Autodesk Inventor part; units mm, degrees
ref_plane "YZ Plane" through (0, 0, 0) normal (1, 0, 0) x (0, 1, 0)
ref_plane "XZ Plane" through (0, 0, 0) normal (0, 1, 0) x (-1, 0, 0)
ref_plane "XY Plane" through (0, 0, 0) normal (0, 0, 1) x (1, 0, 0)
sketch "Sketch1" plane through (0, 0, 0) normal (0, 1, 0) x (-1, 0, 0)
  line L0 (5.3777, 6.5934) -> (5.3777, -88.6566)
  line L1 (5.3777, -88.6566) -> (-39.0723, -88.6566)
  line L2 (-39.0723, -88.6566) -> (-39.0723, 6.5934)
  line L3 (-39.0723, 6.5934) -> (5.3777, 6.5934)
  point P0 (0, 0)
  dimension "d0" = 95.25
  dimension "d1" = 44.45
extrude "Extrusion1" add sketch "Sketch1" along normal blind 3.175
sketch "Sketch2" plane through (0, 3.175, 0) normal (0, 1, 0) x (1, 0, 0)
  line L0 (39.0723, 88.6566) -> (-5.3777, 88.6566)
  line L1 (-5.3777, 88.6566) -> (-2.2027, 88.6566)
  line L2 (-2.2027, 88.6566) -> (-2.2027, 85.4816)
  line L3 (-2.2027, 85.4816) -> (-1.9487, 85.4816)
  line L4 (-1.9487, 85.4816) -> (-1.9487, 49.9216)
  line L5 (-1.9487, 49.9216) -> (-2.2027, 49.9216)
  line L6 (-2.2027, 49.9216) -> (-2.2027, 85.4816)
  point P0 (0, 0)
  dimension "d4" = 3.175
  dimension "d5" = 3.175
  dimension "d6" = 0.254
  dimension "d7" = 35.56
  dimension "d8" = 35.56
extrude "Extrusion2" add sketch "Sketch2" along normal blind 0.254
fillet "Fillet1" radius 0.127 2 edges at (-1.9487, 3.429, -67.7016) (-2.2027, 3.429, -67.7016)
sketch "Sketch3" plane through (0, 3.175, 0) normal (0, 1, 0) x (1, 0, 0)
  line L0 (39.0723, -6.5934) -> (39.0723, 88.6566)
  line L1 (39.0723, 88.6566) -> (35.9091, 88.6566)
  line L2 (39.0723, 88.6566) -> (-5.3777, 88.6566)
  line L3 (35.9091, 88.6566) -> (35.9091, 85.4816)
  line L4 (35.9091, 85.4816) -> (35.6551, 85.4816)
  line L5 (35.6551, 85.4816) -> (35.6551, 49.9216)
  line L6 (35.6551, 49.9216) -> (35.9091, 49.9216)
  line L7 (35.9091, 49.9216) -> (35.9091, 85.4816)
  point P0 (0, 0)
  dimension "d12" = 3.175
  dimension "d13" = 0.254
  dimension "d14" = 35.56
  dimension "d15" = 0.254
  dimension "d16" = 35.56
extrude "Extrusion3" add sketch "Sketch3" along normal blind 0.254
fillet "Fillet2" radius 0.127 2 edges at (35.9091, 3.429, -67.7016) (35.6551, 3.429, -67.7016)
sketch "Sketch4" plane through (0, 3.175, 0) normal (0, 1, 0) x (1, 0, 0)
  line L0 (-1.9487, 85.4816) -> (-1.9487, 49.9216)
  line L1 (35.6551, 49.9216) -> (35.6551, 85.4816)
  line L2 (-1.9487, 85.4816) -> (35.6551, 85.4816)
  line L3 (35.6551, 85.4816) -> (35.6551, 85.2276)
  line L4 (35.6551, 85.2276) -> (-1.9487, 85.2276)
  line L5 (-1.9487, 85.2276) -> (-1.9487, 85.4816)
  point P0 (0, 0)
  dimension "d20" = 0.254
extrude "Extrusion4" add sketch "Sketch4" along normal blind 0.254
fillet "Fillet3" radius 0.127 2 edges at (16.8532, 3.429, -85.2276) (16.8532, 3.429, -85.4816)
sketch "Sketch5" plane through (-2.2027, 3.175, -85.4816) normal (-1, 0, 0) x (0, 0, 1)
  point P0 (85.4816, -3.175)
sketch "Sketch6" plane through (0, 3.175, 0) normal (0, 1, 0) x (1, 0, 0)
  line L0 (-2.2027, 85.4816) -> (-1.9487, 85.4816)
  line L1 (-2.2027, 85.4816) -> (-2.4567, 85.4816)
  line L2 (35.6551, 85.4816) -> (-1.9487, 85.4816)
  line L3 (-1.9487, 85.4816) -> (-1.6947, 85.4816)
  line L4 (-1.6947, 85.4816) -> (-1.6947, 117.2316)
  line L5 (-2.2027, 85.4816) -> (-2.2027, 117.2316)
  line L6 (-2.2027, 117.2316) -> (-1.6947, 117.2316)
  point P0 (0, 0)
  dimension "d24" = 0.254
  dimension "d25" = 0.254
  dimension "d26" = 31.75
extrude "Extrusion5" add sketch "Sketch6" along normal blind 0.508
fillet "Fillet4" radius 0.127 1 edges at (-1.9487, 3.683, -85.4816)
sketch "Sketch7" plane through (0, 3.683, 0) normal (0, 1, 0) x (1, 0, 0)
  line L0 (-2.2027, 117.2316) -> (-2.2027, 88.6566)
  line L1 (-2.2027, 117.2316) -> (-2.2027, 114.0566)
  line L2 (-2.2027, 114.0566) -> (-1.6947, 114.0566)
  line L3 (-1.6947, 85.6086) -> (-1.6947, 117.2316)
  line L4 (-2.2027, 114.0566) -> (-2.2027, 113.8026)
  line L5 (-2.2027, 113.8026) -> (-1.6947, 113.8026)
  line L6 (-1.6947, 113.8026) -> (-1.6947, 114.0566)
  point P0 (0, 0)
  dimension "d30" = 3.175
  dimension "d31" = 0.254
extrude "Extrusion6" cut sketch "Sketch7" against normal blind 0.254
sketch "Sketch8" plane through (0, 3.683, 0) normal (0, 1, 0) x (1, 0, 0)
  line L0 (-1.6947, 113.8026) -> (-2.2027, 113.8026)
  line L1 (-2.2027, 113.8026) -> (-2.2027, 107.4526)
  line L2 (-2.2027, 117.2316) -> (-2.2027, 88.6566)
  line L3 (-2.2027, 107.4526) -> (-1.6947, 107.4526)
  line L4 (-1.6947, 88.6566) -> (-1.6947, 117.2316)
  line L5 (-2.2027, 107.4526) -> (-2.2027, 107.1986)
  line L6 (-2.2027, 107.1986) -> (-1.6947, 107.1986)
  line L7 (-1.6947, 107.4526) -> (-1.6947, 107.1986)
  line L8 (-2.2027, 107.4526) -> (-1.6947, 107.4526)
  line L9 (-1.6947, 107.1986) -> (-1.6947, 107.4526)
  line L10 (-2.2027, 107.4526) -> (-2.2027, 107.1986)
  line L11 (-2.2027, 107.1986) -> (-1.6947, 107.1986)
  point P0 (0, 0)
  dimension "d34" = 6.35
  dimension "d35" = 0.254
extrude "Extrusion7" cut sketch "Sketch8" against normal blind 0.254 contours L4 L6 L2 L3
sketch "Sketch9" plane through (0, 3.175, 0) normal (0, 1, 0) x (1, 0, 0)
  line L0 (-2.2027, 85.4816) -> (-2.2027, 49.9216)
  line L1 (35.9091, 49.9216) -> (35.6551, 49.9216)
  line L2 (-2.2027, 49.9216) -> (35.9091, 49.9216)
  line L3 (35.9091, 49.9216) -> (35.9091, 47.3816)
  line L4 (35.9091, 47.3816) -> (-2.2027, 47.3816)
  line L5 (-2.2027, 47.3816) -> (-2.2027, 49.9216)
  point P0 (0, 0)
  dimension "d38" = 2.54
extrude "Extrusion8" add sketch "Sketch9" along normal blind 1.27
fillet "Fillet5" radius 0.254 2 edges at (16.8532, 4.445, -47.3816) (16.8532, 4.445, -49.9216)
properties part number "mousetrap"
Geometry check sheet. Reference: the model listing, model coordinates, mm. Give positions to 0.01 mm unless a question says otherwise; leave off trailing zeros. Loops run counter-clockwise (first coordinate to the right, second up) from the corner with the lowest first, then second, coordinate; pieces in that order, holes last. Notation, with made-up numbers: M -12.75,-8 L 41.25,-8 A12 cw 41.25,2 Z; hole C 76,20.5 d5. An arc over 180 degrees is marked long. Answer as CSV lines item,"result".
Item 1: Cross-section at D-D on z = -13.5. Record the cut outline in (x, y) (3 decimals).
Values:
outline,"M -5.378,0 L 39.072,0 L 39.072,3.175 L -5.378,3.175 Z"
Item 2: Material ranges on line 1 (Y direction, x = 8, z = -25.5) (3 decimals); line 2 (Z direction, x = 17, y = 1.3); line 3 (X direction, y = 3.35, z = -103.5), recorded low to high.
Values:
line 1,"y = 0 to 3.175"
line 2,"z = -88.66 to 6.59"
line 3,"x = -2.2 to -1.69"
Item 3: Release check for a two-part mould opening along Z. For faces 1 (the flat face through (17, 3.175, -67)), 2 (the flat face through (-5.378, 2, -40)), 3 (the flat face through (17, 2, -88.657)) record: pulls with the +Z half, pulls with the -Z half, needs draft (parallel to the pull), parting line crosses it, or undercut.
Values:
face 1,"undercut"
face 2,"needs draft"
face 3,"pulls with the -Z half"
Item 4: Cross-section at C-C on y = 2. Record the cut outline in (x, z), and give its area (3 significant figures).
Values:
outline,"M -5.38,-88.66 L 39.07,-88.66 L 39.07,6.59 L -5.38,6.59 Z"
area,"4,230 mm²"
Item 5: Cross-section at B-B on x = 7.5. Record the cut outline in (y, z) (3 decimals).
Values:
outline,"M 0,-88.657 L 3.175,-88.657 L 3.175,-85.482 L 3.305,-85.482 A0.124 ccw 3.429,-85.358 L 3.429,-85.352 A0.124 ccw 3.305,-85.228 L 3.175,-85.228 L 3.175,-49.922 L 4.191,-49.922 A0.254 ccw 4.445,-49.668 L 4.445,-47.636 A0.254 ccw 4.191,-47.382 L 3.175,-47.382 L 3.175,6.593 L 0,6.593 Z"
Item 6: Depth check by flat-ended pin: P1, Ø5, axis at x = -0.5, z = -69, coming from the +Y side; P2, Ø8, axis at x = 20.5, z = -81, coming from the +Y side (3 decimals); P3, Ø1.4, axis at y = 4, z = -67.5, coming from the +X side. Enter the tip coordinate at first touch or a pass-through.
Values:
P1,"stops at y = 3.43"
P2,"stops at y = 3.175"
P3,"stops at x = 35.91"
